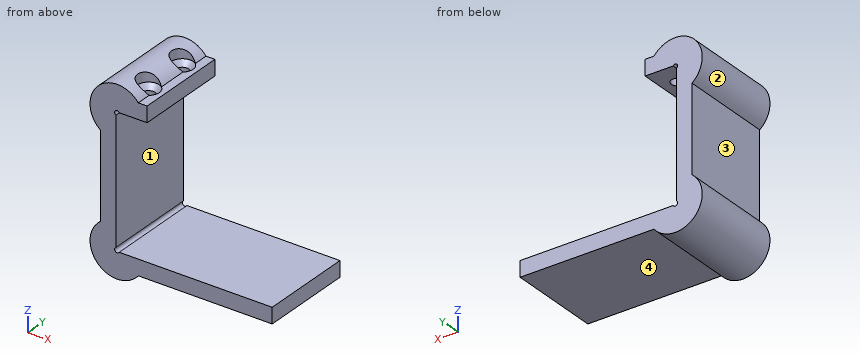
Autodesk Fusion 360 part; units mm, degrees
sketch "Sketch1" plane through (0, 0, 0) normal (0, 1, 0) x (1, 0, 0)
  line L0 (0, 0) -> (0, 53)
  line L1 (0, 0) -> (12.7, 0)
  line L2 (0, 53) -> (63.5, 53)
  line L3 (-6.35, 59.35) -> (63.5, 59.35)
  line L4 (-6.35, -6.35) -> (-6.35, 59.35)
  line L5 (-6.35, -6.35) -> (12.7, -6.35)
  line L6 (12.7, -6.35) -> (12.7, 0)
  line L7 (63.5, 53) -> (63.5, 59.35)
  line L8 (-6.35, -6.35) -> (0.5, 0.5) construction
  line L9 (-6.35, 59.35) -> (0.5, 52.5) construction
  dimension "d1" = 53
  dimension "d2" = 12.7
  dimension "d3" = 63.5
  dimension "d5" = 6.35
  dimension "d6" = 0.5
  dimension "d7" = 0.5
sketch "Sketch2" plane through (0, 0, 0) normal (0, 1, 0) x (1, 0, 0)
  circle A0 centre (0.5, 0.5) radius 1
  circle A1 centre (0.5, 52.5) radius 1
  circle A2 centre (0.5, 52.5) radius 11
  line L0 (-6.35, -6.35) -> (-6.35, 59.35)
  line L1 (-6.35, 59.35) -> (63.5, 59.35)
  line L2 (-6.35, -6.35) -> (12.7, -6.35)
  circle A3 centre (0.5, 0.5) radius 11
  point P0 (0.5, 0.5)
  point P1 (0.5, 52.5)
  dimension "d8" = 2
  dimension "d9" = 22
ref_plane "WorkPlane1" through (0, 0, 6.35) normal (0, 0, 1) x (1, 0, 0)
sketch "Sketch3" plane through (0, 0, 6.35) normal (0, 0, 1) x (1, 0, 0)
  line L0 (-6.35, 0) -> (12.7, 0)
  line L1 (-6.35, 0) -> (12.7, 0) construction
  line L2 (12.7, 0) -> (12.7, 38.1)
  line L3 (12.7, 38.1) -> (-6.35, 38.1)
  line L4 (-6.35, 38.1) -> (-6.35, 0)
  line L5 (6.35, 0) -> (6.35, 38.1) construction
  line L6 (12.7, 19.05) -> (6.35, 19.05) construction
  circle A0 centre (6.35, 28.575) radius 4.4196
  circle A1 centre (6.35, 9.525) radius 4.4196
  line L7 (0, 0) -> (12.7, 0)
  point P0 (6.35, 9.525)
  point P1 (6.35, 28.575)
  dimension "d11" = 38.1
  dimension "d12" = 19.05
  dimension "d13" = 8.8392
extrude "Extrude1" add sketch "Sketch1" along normal up to surface (38.1 mm away)
extrude "Extrude2" add sketch "Sketch2" along normal up to surface (38.1 mm away) contours L0 L2 A3 | A2 L0 L1 picked at (-6.7442, 3.5907) picked at (-6.7442, 49.4093)
extrude "Extrude3" cut sketch "Sketch3" along normal blind 5 contours A0 | A1
hole "Hole1" at (6.35, 28.575, 6.35) at (6.35, 9.525, 6.35) direction (0, 0, -1) diameter 5.08 depth 25 tip angle 118 countersink diameter 8.8392 countersink angle 82
extrude "Extrude4" cut sketch "Sketch2" along normal up to surface (38.1 mm away) contours A0 | A1
equation "d2 = ( 0.5 * 25.4 ) * 1 mm"
equation "d3 = ( 2.5 * 25.4 ) * 1 mm"
equation "d11 = ( 1.5 * 25.4 ) * 1 mm"
equation "d12 = ( 0.75 * 25.4 ) * 1 mm"
Read the model definition and answer for the solid it produces. Units are mm, in the model's axes. Face numbers are marked on the shaded views. A direction names the side the tool comes from. Coordinates: 2 decimals unless noted, no trailing zeros. Loops run counter-clockwise (first coordinate to the right, second up) from the corner with the lowest first, then second, coordinate; pieces in that order, holes last.
Q1. The part is cut by section A-A on y = 34. Write down the section's boundary in (x, z).
Q2. The part is cut by section D-D on z = -32. Write down the section's boundary in (x, y).
Q3. Each of these flat-tipped pins is pushed along its axis until it touches: pin 1 Ø1 at (y, z) = (15.5, -51) entering from +X; pin 2 Ø10 at (x, y) = (6.35, 28.575) entering from +Z; pin 3 Ø12 at (x, y) = (54.5, 34) entering from -Z. Where does it stop, or does it pass through?
Q4. Consider probe 1 along Y at (x, z) = (6.35, 3.2) (3 decimals); probe 2 along Y at (x, z) = (6.35, 8.3); probe 3 along Z at (x, y) = (12, 32). Determine where each line is inside the solid, lowest interval first.
Q5. The part is cut by section B-B on x = 6.35. Write down the section's boundary in (y, z) (3 decimals).
Q6. The part is cut by section C-C on x = 45.5. Write down the section's boundary in (y, z).
Q7. Which of the six approach directions +Z, -Z, +X, -X, +Y, -Y give full straight-line access (tool end or side, diameter ignored) to the marked faces 1, 2, 3 and 4?
Results below:
1. outline: (-6.35, -43.89) arc R11 ccw (long way) to (9.11, -59.35) - (63.5, -59.35) - (63.5, -53) - (1.37, -53) arc R1 cw (long way) to (0, -51.63) - (0, -1.37) arc R1 cw (long way) to (1.37, 0) - (12.7, 0) - (12.7, 6.35) - (9.11, 6.35) arc R11 ccw (long way) to (-6.35, -9.11) - close
2. outline: (-6.35, 0) - (0, 0) - (0, 38.1) - (-6.35, 38.1) - close
3. pin 1: stops at x = 0
3. pin 2: stops at z = 10.47
3. pin 3: stops at z = -59.35
4. probe 1: y = 0 to 6.985, 12.065 to 26.035, 31.115 to 38.1
4. probe 2: y = 0 to 5.11, 13.94 to 24.16, 32.99 to 38.1
4. probe 3: z = -59.35 to -53, 0 to 6.35
5. outline: (0, -61.815) - (38.1, -61.815) - (38.1, -53) - (0, -53) - close; (0, 0) - (6.985, 0) - (6.985, 4.188) - (5.105, 6.35) - (5.105, 8.815) - (0, 8.815) - close; (12.065, 0) - (26.035, 0) - (26.035, 4.188) - (24.155, 6.35) - (24.155, 8.815) - (13.945, 8.815) - (13.945, 6.35) - (12.065, 4.188) - close; (31.115, 0) - (38.1, 0) - (38.1, 8.815) - (32.995, 8.815) - (32.995, 6.35) - (31.115, 4.188) - close
6. outline: (0, -59.35) - (38.1, -59.35) - (38.1, -53) - (0, -53) - close
7. face 1: +X, +Y, -Y
7. face 2: +Y, -Y
7. face 3: -X, +Y, -Y
7. face 4: -Z, +X, +Y, -Y
